CAD build for the part. Positions are in the model's coordinates, mm. A direction names the side the tool comes from. Coordinates: 2 decimals unless noted, no trailing zeros. Loops run counter-clockwise (first coordinate to the right, second up) from the corner with the lowest first, then second, coordinate; pieces in that order, holes last. Notation, with made-up numbers: (10, 7) -> (69, 7) arc R21 cw to (69, 21) -> close; hole circle Ø5 at (4, 14.25). An arc over 180 degrees is marked (long way). Write item = value, one per line. Start each with the question number.
(1) Band-saw the part on D-D (x = 19). Write the cut outline in (y, z) (3 decimals).
(2) Flat gauge pins, fed straight in: P1, Ø1.9, axis at x = 17, y = -4.5, coming from the +Z side (3 decimals); P2, Ø1.5, axis at x = 16, z = 50.5, coming from the +Y side (3 decimals); P3, Ø5, axis at x = 22, y = -2, coming from the -Z side (3 decimals); P4, Ø5.5, axis at y = 12.7, z = 101.6, coming from the +X side. Where does each tip first touch, or does it go through?
(3) Pull direction Z, two halves, no side cores. Call faces 4 (the face through (30.18, 11.48, 149.47)), 5 (the face through (30, 10, 190.5)), 6 (the face through (1.91, -4.54, 93.92)), 7 (the face through (1.61, 12.84, 180.97)): +Z half, -Z half, draft (parallel to the pull), parting line (faces both ways), or undercut.
(4) Band-saw the part on C-C (z = 101.6). Write the cut outline in (x, y) (3 decimals), and give its area (3 significant figures).
(5) Tool access for faces 1 (the face through (2, 10, 190.5)), 2 (the face through (16, -5, 28.575)), 3 (the face through (4.13, -2.27, 94.32)): list every direction of +Z, -Z, +X, -X, +Y, -Y with a clear straight run to the whole face (end or side of a thin tool).
(6) Drill centre lines: line 1 (Y direction, x = 30.9, z = 152.4) (3 decimals); line 2 (X direction, y = 3.5, z = 100) (3 decimals); line 3 (Y direction, x = 22, z = 135.5) (3 decimals). Where is each one in solid material? Low to high. Write a range as from..to.
(7) Band-saw the part on B-B (y = 7.5). Write the cut outline in (x, z) (3 decimals).
(8) Band-saw the part on A-A (z = 25.4). Write the cut outline in (x, y) (3 decimals).
Autodesk Inventor part; units mm, degrees
ref_plane "YZ Plane" through (0, 0, 0) normal (1, 0, 0) x (0, 1, 0)
ref_plane "XZ Plane" through (0, 0, 0) normal (0, 1, 0) x (-1, 0, 0)
ref_plane "XY Plane" through (0, 0, 0) normal (0, 0, 1) x (1, 0, 0)
sketch "Sketch1" plane through (0, 0, 0) normal (0, 0, 1) x (1, 0, 0)
  line L0 (0, 25.4) -> (0, 0)
  line L1 (6.35, -6.35) -> (25.4, -6.35)
  line L2 (31.75, 0) -> (31.75, 25.4)
  line L3 (31.75, 25.4) -> (28.575, 25.4)
  line L4 (28.575, 25.4) -> (28.575, 0)
  line L5 (25.4, -3.175) -> (6.35, -3.175)
  line L6 (3.175, 0) -> (3.175, 25.4)
  line L7 (3.175, 25.4) -> (0, 25.4)
  arc A0 (3.175, 0) -> (6.35, -3.175) centre (6.35, 0) ccw
  arc A1 (0, 0) -> (6.35, -6.35) centre (6.35, 0) ccw
  arc A2 (25.4, -3.175) -> (28.575, 0) centre (25.4, 0) ccw
  arc A3 (25.4, -6.35) -> (31.75, 0) centre (25.4, 0) ccw
  dimension "d0" = 3.175
  dimension "d1" = 25.4
  dimension "d2" = 25.4
  dimension "d3" = 3.175
extrude "Extrusion1" add sketch "Sketch1" along normal blind 190.5
sketch "Sketch2" plane through (31.75, 0, 0) normal (1, 0, 0) x (0, 0, -1)
  line L0 (-190.5, 25.4) -> (-190.5, 0)
  line L1 (0, 25.4) -> (-190.5, 25.4)
  circle A0 centre (-177.8, 12.7) radius 3.175
  dimension "d6" = 6.35
  dimension "d7" = 12.7
  dimension "d8" = 12.7
extrude "Extrusion2" cut sketch "Sketch2" against normal through all
pattern_linear "Rectangular Pattern1" count 7 spacing 25.4 along (0, 0, -1) of "Extrusion2"
sketch "Sketch3" plane through (6.35, -6.35, 0) normal (0, -1, 0) x (1, 0, 0)
  line L0 (19.05, 190.5) -> (0, 190.5)
  circle A0 centre (9.525, 139.7) radius 6.35
  point P0 (-6.35, 0)
  dimension "d14" = 12.7
  dimension "d15" = 50.8
extrude "Extrusion3" cut sketch "Sketch3" against normal up to next
sketch "Sketch4" plane through (6.35, -6.35, 0) normal (0, -1, 0) x (1, 0, 0)
  line L0 (19.05, 190.5) -> (0, 190.5)
  line L1 (0, 0) -> (0, 190.5)
  line L2 (0, 0) -> (19.05, 0)
  line L3 (19.05, 0) -> (19.05, 190.5)
  line L4 (-3.175, 190.5) -> (22.225, 190.5)
  line L5 (22.225, 190.5) -> (22.225, 161.925)
  line L6 (22.225, 161.925) -> (-3.175, 161.925)
  line L7 (-3.175, 161.925) -> (-3.175, 190.5)
  line L8 (-3.175, 165.9576) -> (0, 165.9576) construction
  line L9 (19.05, 165.9576) -> (22.225, 165.9576) construction
  line L10 (-3.175, 0) -> (22.225, 0)
  line L11 (22.225, 0) -> (22.225, 28.575)
  line L12 (22.225, 28.575) -> (-3.175, 28.575)
  line L13 (-3.175, 28.575) -> (-3.175, 0)
  line L14 (-6.35, 190.5) -> (-3.175, 190.5)
  line L15 (-3.175, 190.5) -> (-3.175, 161.925)
  line L16 (-3.175, 161.925) -> (-6.35, 161.925)
  line L17 (-6.35, 161.925) -> (-6.35, 190.5)
  point P0 (-6.35, 0)
  dimension "d18" = 25.4
  dimension "d19" = 28.575
  dimension "d20" = 0
  dimension "d21" = 0
extrude "Extrusion4" cut sketch "Sketch4" against normal through all contours L3 L6 L1 L0 | L4 L5 L6 L3 | L1 L6 L7 L4 | L12 L11 L10 L3 | L3 L2 L1 L12 | L1 L10 L13 L12
properties part number "Frame_OuterConveyorMount" material "Aluminum-6061"
Findings below:
q1.outline = (-6.35, 28.575) -> (-3.175, 28.575) -> (-3.175, 134.172) -> (-6.35, 134.172) -> close; (-6.35, 145.228) -> (-3.175, 145.228) -> (-3.175, 161.925) -> (-6.35, 161.925) -> close
q2.P1 = 161.925
q2.P2 = -3.175
q2.P3 = 28.575
q2.P4 = through
q3.face_4 = undercut
q3.face_5 = +Z half
q3.face_6 = draft
q3.face_7 = undercut
q4.outline = (0, 0) arc R6.35 ccw to (6.35, -6.35) -> (25.4, -6.35) arc R6.35 ccw to (31.75, 0) -> (31.75, 9.525) -> (28.575, 9.525) -> (28.575, 0) arc R3.175 cw to (25.4, -3.175) -> (6.35, -3.175) arc R3.175 cw to (3.175, 0) -> (3.175, 9.525) -> (0, 9.525) -> close; (0, 15.875) -> (3.175, 15.875) -> (3.175, 25.4) -> (0, 25.4) -> close; (28.575, 15.875) -> (31.75, 15.875) -> (31.75, 25.4) -> (28.575, 25.4) -> close
q4.area = 229 mm²
q5.face_1 = +Z, +X, -X, +Y, -Y
q5.face_2 = -Z, +Y, -Y
q5.face_3 = +Z, -Z, +Y
q6.line_1 = -3.174..9.525, 15.875..25.4
q6.line_2 = 0..3.175, 28.575..31.75
q6.line_3 = -6.35..-3.175
q7.outline = (0, 0) -> (3.175, 0) -> (3.175, 190.5) -> (0, 190.5) -> close; (28.575, 0) -> (31.75, 0) -> (31.75, 190.5) -> (28.575, 190.5) -> close
q8.outline = (0, 0) arc R6.35 ccw to (3.175, -5.499) -> (3.175, 9.525) -> (0, 9.525) -> close; (0, 15.875) -> (3.175, 15.875) -> (3.175, 25.4) -> (0, 25.4) -> close; (28.575, -5.499) arc R6.35 ccw to (31.75, 0) -> (31.75, 9.525) -> (28.575, 9.525) -> close; (28.575, 15.875) -> (31.75, 15.875) -> (31.75, 25.4) -> (28.575, 25.4) -> close
